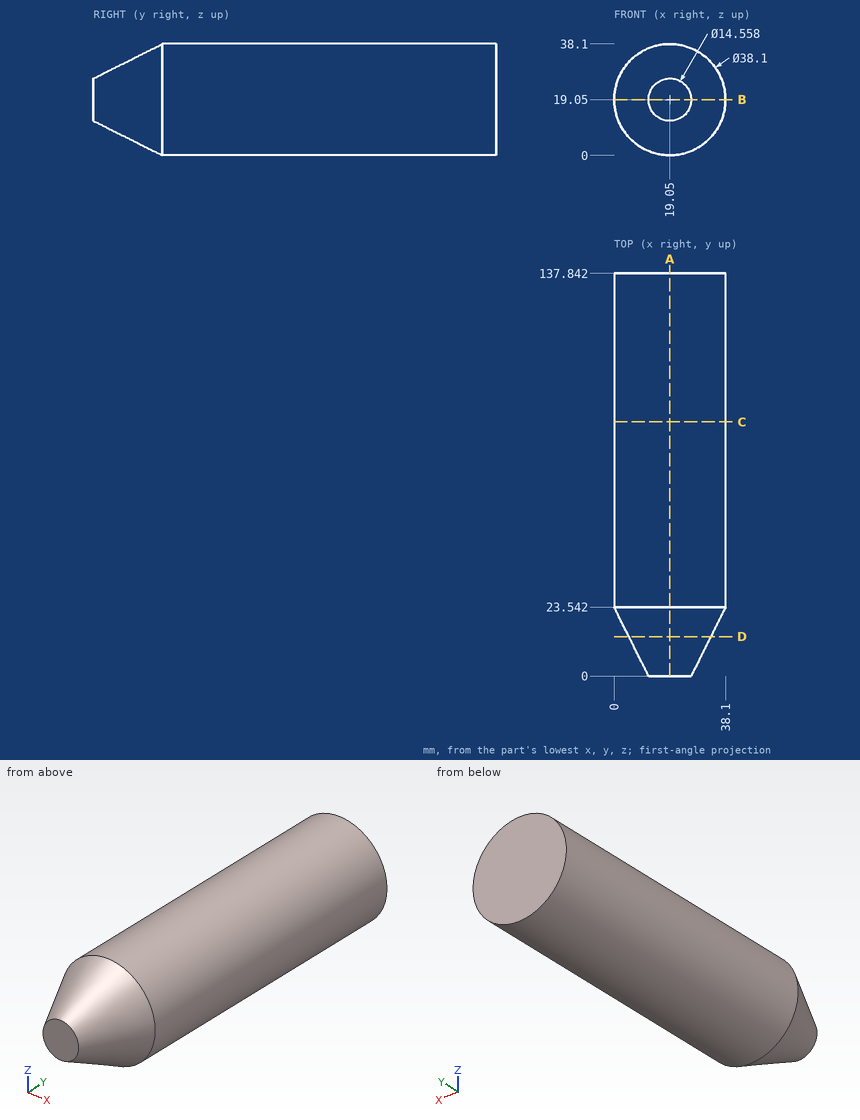
Print and shaded views of the part. All mm, measured from the part's lowest x, y and z. Coordinates: 2 decimals unless noted, no trailing zeros. Loops run counter-clockwise (first coordinate to the right, second up) from the corner with the lowest first, then second, coordinate; pieces in that order, holes last. Notation, with made-up numbers: (87, 38) - (128, 38) arc R11 cw to (128, 48) - close; hole circle Ø11 at (45.5, -4.5). An arc over 180 degrees is marked (long way). Use one line per item in the form item = value. Start each with the question number.
1) Band-saw the part on C-C (y = 87). Give the cut face in (x, z), and give its area (3 significant figures).
2) Drill centre lines: L1, parallel to Z at x = 19, y = 80; L2, parallel to X at y = 57, z = 6; L3, parallel to X at y = 47.5, z = 4. Where is each one in solid material? Low to high. Write a range as from..to.
3) Band-saw the part on B-B (z = 19.05). Give the cut face in (x, y).
4) Flat gauge pins, fed straight in: pin 1 (12 mm diameter, centred on y = 116, z = 31, fed in from -X); pin 2 (5 mm diameter, centred on x = 19.5, y = 115.5, fed in from -Z); pin 3 (2 mm diameter, centred on x = 15.5, y = 49.5, fed in from +Z). Where does each tip first touch, or does it go through?
5) Band-saw the part on A-A (x = 19.05). Give the cut face in (y, z).
6) Band-saw the part on D-D (y = 13.5). Give the cut face in (x, z).
Check values:
q1.outline = circle Ø38.1 at (19.05, 19.05)
q1.area = 1,140 mm2
q2.L1 = 0..38.1
q2.L2 = 5.17..32.93
q2.L3 = 7.37..30.73
q3.outline = (0, 23.54) - (11.77, 0) - (26.33, 0) - (38.1, 23.54) - (38.1, 137.84) - (0, 137.84) - close
q4.pin_1 = 0.95
q4.pin_2 = 0
q4.pin_3 = 37.93
q5.outline = (0, 11.77) - (23.54, 0) - (137.84, 0) - (137.84, 38.1) - (23.54, 38.1) - (0, 26.33) - close
q6.outline = circle Ø28.06 at (19.05, 19.05)
